```python
from build123d import *

# Parameters (mm, degrees)
F0_R     = 9.8592181747
F1_DEPTH = 2
F2_R     = 5
F3_DEPTH = 0.5
F4_R     = 4.05
F5_DEPTH = 3.3
F6_R     = 8.5
F7_DEPTH = 1


# Not quite as in the source:
# - a fillet or chamfer that OpenCascade refuses, or shapes differently, is made with other operations: its cross-section is extruded or revolved along the edge and cut away or added


with BuildPart() as f1:
    # F0 (on Top) → F1 (new body)
    with BuildSketch(Plane.XY):
        Circle(F0_R)
    extrude(amount=F1_DEPTH)

    # F2 (on face) → F3 (join)
    with BuildSketch(Plane.XY.offset(2)):
        Circle(F2_R)
    extrude(amount=F3_DEPTH)

    # F4 (on face) → F5 (join)
    with BuildSketch(Plane.XY.offset(2.5)):
        Circle(F4_R)
    extrude(amount=F5_DEPTH)

    # F6 (on face) → F7 (cut)
    with BuildSketch(Plane(origin=(0, 0, 0), x_dir=(1, 0, 0), z_dir=(0, 0, -1))):
        Circle(F6_R)
    extrude(amount=-F7_DEPTH, mode=Mode.SUBTRACT)

    # F8: fillet of radius 32 on 1 edges, made by hand

    # F8_s1 → F8_t2 (revolve)
    with BuildSketch(Plane.XZ):
        with BuildLine():
            ThreePointArc((8.5, 0), (4.5627460668, 0.7490157328), (0.5627460668, 1))
            Line((0.5627460668, 1), (8.5, 1))
            Line((8.5, 1), (8.5, 0))
        make_face()
    revolve(axis=Axis((0, 0, 1), (0, 0, -1)))

    # F9: fillet of radius 1.5 on 1 edges, made by hand

    # F9_s1 → F9_t2 (revolve, cut)
    with BuildSketch(Plane.XZ):
        with BuildLine():
            ThreePointArc((9.8592181747, 1.4933788795), (9.4685361494, 0.4837187233), (8.5, 0))
            Line((8.5, 0), (9.8592181747, 0))
            Line((9.8592181747, 0), (9.8592181747, 1.4933788795))
        make_face()
    revolve(axis=Axis((0, 0, 0), (0, 0, 1)), mode=Mode.SUBTRACT)


solid = f1.part
```
Source: CAD feature listing. Evaluate the final solid. Frame: model axes, mm. A direction names the side the tool comes from. Round coordinates to 2 decimals unless told otherwise and drop trailing zeros. Order: outer loops, then holes, each group sorted by start corner. A loop starts at its lowest first (then second) coordinate and runs counter-clockwise, first axis right, second up. Notation, with made-up numbers: (30.5, -31.75) -> (63.5, -31.75) arc R22 cw to (63.5, -8.75) -> close; hole circle Ø9 at (26, -7.75). An arc over 180 degrees is marked (long way). Use CSV: the item, a comma, the result in double quotes.
(1) First-contact query: pin 1 Ø1 at (y, z) = (-2.5, 0.5) entering from -X; pin 2 Ø1.2 at (x, y) = (0, 0) entering from -Z; pin 3 Ø3 at (y, z) = (6.5, 1) entering from -X. Flat tips, straight axial feed; report the tip coordinate or a pass-through.
Report:
pin 1,"x = -9.49"
pin 2,"z = 1"
pin 3,"x = -8.47"
(2) Section A-A on z = 3.7. Return the cut outline in (x, y).
Report:
outline,"circle Ø8.1 at (0, 0)"
(3) Access query for faces 1 (the face through (-1.08, -4.88, 2.25)), 2 (the face through (0, 0, 1)), 3 (the face through (0, 0, 5.8)). Directions: +Z, -Z, +X, -X, +Y, -Y. A direction counts if a zero-diameter tool reaches every point of the face in a straight line with its end or side. Return the directions, or none.
Report:
face 1,"+Z"
face 2,"-Z"
face 3,"+Z, +X, -X, +Y, -Y"
(4) Ray query, L1, parallel to Z at x = 0.5, y = 0.5; L2, parallel to X at y = -7.5, z = 1.7; L3, parallel to Y at x = -3, z = 5.25. Return the intervals inside material, ascending.
Report:
L1,"1 to 5.8"
L2,"-6.4 to 6.4"
L3,"-2.72 to 2.72"
